Part model, mm, in its own coordinate system. Round coordinates to 2 decimals unless told otherwise and drop trailing zeros. Order: outer loops, then holes, each group sorted by start corner. A loop starts at its lowest first (then second) coordinate and runs counter-clockwise, first axis right, second up. Notation, with made-up numbers: M -33,-12 L -19,-12 A15 cw -19,14 Z; hole C 71,25.5 d11. An arc over 180 degrees is marked long. One line per question, with ' | ' between items.
from build123d import *

# Parameters (mm, degrees)
F_7_0_201_DIAMETER_HOLE1_D     = 5.1054
F_7_0_201_DIAMETER_HOLE1_DEPTH = 101.176865362
CIRPATTERN1_COUNT              = 3
SKETCH7_R                      = 2.54
CUT_EXTRUDE1_DEPTH             = 84.368801521


with BuildPart() as part:
    # Sketch1 one side → Revolve1 (revolve)
    with BuildSketch(Plane.XY, mode=Mode.PRIVATE) as revolve1_sk:
        with BuildLine():
            ThreePointArc((0, -38.608), (-33.727527511, -18.789133881), (-32.827964664, 20.32))
            Line((-32.827964664, 20.32), (-44.338235562, 18.7325))
            ThreePointArc((-44.338235562, 18.7325), (-40.115066443, -26.600134083), (0, -48.133))
            Line((0, -48.133), (0, -38.608))
        make_face()
    revolve(revolve1_sk.sketch.rotate(Axis((0, 48.133, 0), (0, -1, 0)), 180), axis=Axis((0, 48.133, 0), (0, -1, 0)))

    # #7 (0.201) Diameter Hole1
    with Locations(Plane(origin=(-36.176279369, -31.75, 0), x_dir=(0.65963060686, -0.751589956355, 0), z_dir=(-0.751589956355, -0.65963060686, 0))):
        with Locations((0, 0)):
            f_7_0_201_diameter_hole1 = Hole(F_7_0_201_DIAMETER_HOLE1_D / 2, depth=F_7_0_201_DIAMETER_HOLE1_DEPTH)

    # CirPattern1: #7 (0.201) Diameter Hole1 ×3 about axis
    cirpattern1_axis = Axis((0, 18.7325, 0), (0, 1, 0))
    for i in range(1, CIRPATTERN1_COUNT):
        add(f_7_0_201_diameter_hole1.rotate(cirpattern1_axis, i * 360 / CIRPATTERN1_COUNT), mode=Mode.SUBTRACT)

    # Sketch7 → Cut-Extrude1 (cut, through all)
    with BuildSketch(Plane(origin=(0, 0, 0), x_dir=(1, 0, 0), z_dir=(0, 1, 0))):
        with Locations(Location((0, 0, 0), (0, 0, 270))):
            Circle(SKETCH7_R)
    extrude(amount=-CUT_EXTRUDE1_DEPTH, mode=Mode.SUBTRACT)


solid = part.part
1) Probe line 1 (Z direction, x = 10.5, y = 14.5); line 2 (Y direction, x = 21, z = 26); line 3 (X direction, y = -44.5, z = 0). List the from-to ranges inside material, lowest first. Write a range as [from, to].
The answers:
line 1: z = [-44.68, -34.21], [34.21, 44.68] | line 2: y = [-34.64, -19.33], [19.33, 20.24] | line 3: x = [-18.34, -2.54], [2.54, 18.34]
2) Saw through at B-B (z = 0). List the corners of the cut face in (x, y), plus the area to 3 significant figures.
The answers:
outline: M -44.34,18.73 A48.13 ccw -37.81,-29.79 L -30.64,-23.49 A38.61 cw -32.83,20.32 Z; M -34.44,-33.62 A48.13 ccw -2.54,-48.07 L -2.54,-38.52 A38.61 cw -27.27,-27.33 Z; M 2.54,-48.07 A48.13 ccw 44.34,18.73 L 32.83,20.32 A38.61 cw 2.54,-38.52 Z | area: 1,590 mm²
3) Two-plate mould, pull along X, no slides. Class faces 1 (the face through (15.48, 20.22, -29.76)), 2 (the face through (-34.1, -26.7, 0.8)): released by +X, released by -X, zero draft, split by the parting line, or undercut.
The answers:
face 1: split by the parting line | face 2: undercut
4) Drop flat-ended pins along their axis: pin 1 (10 mm diameter, centred on x = 16.5, y = 1.5, fed in from +Z); pin 2 (2 mm diameter, centred on x = 8.5, z = -38, fed in from -Y); pin 3 (5 mm diameter, centred on x = -8, y = -16, fed in from +Z). Give the stop position or say it passes through.
The answers:
pin 1: stops at z = 46.72 | pin 2: stops at y = -29.62 | pin 3: stops at z = 45.61
5) Saw through at C-C (y = 7.5). List the corners of the cut face in (x, z), plus the area to 3 significant figures.
The answers:
outline: C 0,0 d95.09; hole C 0,0 d75.75 | area: 2,600 mm²
6) Saw through at A-A (x = 0). List the corners of the cut face in (y, z).
The answers:
outline: M -48.07,-2.54 A48.13 ccw 18.73,-44.34 L 20.32,-32.83 A38.61 cw -38.52,-2.54 Z; M -48.07,2.54 L -38.52,2.54 A38.61 cw 20.32,32.83 L 18.73,44.34 A48.13 ccw Z
